```python
from build123d import *

# Parameters (mm, degrees)
BOSS_EXTRUDE1_DEPTH     = 6.35
CUT_EXTRUDE2_DEPTH      = 2.54
CUT_EXTRUDE2_DEPTH_BACK = 127
CUT_EXTRUDE4_DEPTH      = 127
CUT_EXTRUDE4_DEPTH_BACK = 127
CUT_EXTRUDE5_DEPTH      = 127
CUT_EXTRUDE5_DEPTH_BACK = 127


with BuildPart() as part:
    # Sketch1 → Boss-Extrude1 (new body)
    with BuildSketch(Plane.XY):
        Polygon((0, 0), (127, 0), (127, 101.6), (0, 101.6), (-70.692427737, 172.292427737), (-91.896861793, 151.087993682), (-91.896861793, 0), align=None)
    extrude(amount=BOSS_EXTRUDE1_DEPTH)

    # Sketch2 → Cut-Extrude2 (cut, two sides)
    with BuildSketch(Plane(origin=(0, 0, 0), x_dir=(-1, 0, 0), z_dir=(0, 0, -1))) as cut_extrude2_sk:
        Polygon((-61.321024484, 65.678975516), (-25.4, 101.6), (-31.75, 101.6), (-49.710512242, 83.639487758), (-67.671024484, 65.678975516), align=None)
    extrude(amount=CUT_EXTRUDE2_DEPTH, mode=Mode.SUBTRACT)
    extrude(cut_extrude2_sk.sketch, amount=-CUT_EXTRUDE2_DEPTH_BACK, mode=Mode.SUBTRACT)

    # Sketch3 → Cut-Extrude4 (cut, two sides)
    with BuildSketch(Plane(origin=(0, 0, 0), x_dir=(-1, 0, 0), z_dir=(0, 0, -1))) as cut_extrude4_sk:
        Polygon((-88.9, 101.6), (-101.6, 101.6), (-101.6, 98.425), (-96.5327, 98.425), (-96.5327, 85.725), (-93.9673, 85.725), (-93.9673, 98.425), (-88.9, 98.425), align=None)
        Polygon((-57.15, 101.6), (-69.85, 101.6), (-69.85, 98.425), (-64.77, 98.425), (-64.77, 85.725), (-62.23, 85.725), (-62.23, 98.425), (-57.15, 98.425), align=None)
        Polygon((-127, 82.55), (-127, 69.85), (-123.825, 69.85), (-123.825, 74.9173), (-111.125, 74.9173), (-111.125, 77.4827), (-123.825, 77.4827), (-123.825, 82.55), align=None)
        Polygon((-127, 57.15), (-127, 44.45), (-123.825, 44.45), (-123.825, 49.5173), (-111.125, 49.5173), (-111.125, 52.0827), (-123.825, 52.0827), (-123.825, 57.15), align=None)
        Polygon((-127, 31.75), (-127, 25.4), (-127, 19.05), (-123.825, 19.05), (-123.825, 24.1173), (-111.125, 24.1173), (-111.125, 26.6827), (-123.825, 26.6827), (-123.825, 31.75), align=None)
        Polygon((-101.6, 3.302), (-101.6, 0), (-88.9, 0), (-88.9, 3.302), (-93.9673, 3.302), (-93.9673, 16.002), (-96.5327, 16.002), (-96.5327, 3.302), align=None)
        Polygon((-25.4, 3.302), (-25.4, 0), (-12.7, 0), (-12.7, 3.302), (-17.7673, 3.302), (-17.7673, 16.002), (-20.3327, 16.002), (-20.3327, 3.302), align=None)
        Polygon((50.8, 3.302), (50.8, 0), (63.5, 0), (63.5, 3.302), (58.4327, 3.302), (58.4327, 16.002), (55.8673, 16.002), (55.8673, 3.302), align=None)
        Polygon((88.721861793, 31.42199842), (91.896861793, 31.42199842), (91.896861793, 44.12199842), (88.721861793, 44.12199842), (88.721861793, 39.05469842), (76.021861793, 39.05469842), (76.021861793, 36.48929842), (88.721861793, 36.48929842), align=None)
        Polygon((88.721861793, 69.193996841), (91.896861793, 69.193996841), (91.896861793, 81.893996841), (88.721861793, 81.893996841), (88.721861793, 76.826696841), (76.021861793, 76.826696841), (76.021861793, 74.261296841), (88.721861793, 74.261296841), align=None)
        Polygon((88.721861793, 106.965995261), (91.896861793, 106.965995261), (91.896861793, 119.665995261), (88.721861793, 119.665995261), (88.721861793, 114.598695261), (76.021861793, 114.598695261), (76.021861793, 112.033295261), (88.721861793, 112.033295261), align=None)
        Polygon((70.692427737, 158.822043556), (66.202299677, 154.331915495), (63.957235647, 156.576979525), (68.447363707, 161.067107586), align=None)
    extrude(amount=CUT_EXTRUDE4_DEPTH, mode=Mode.SUBTRACT)
    extrude(cut_extrude4_sk.sketch, amount=-CUT_EXTRUDE4_DEPTH_BACK, mode=Mode.SUBTRACT)

    # Sketch4 → Cut-Extrude5 (cut, two sides)
    with BuildSketch(Plane.XY) as cut_extrude5_sk:
        Polygon((-81.917747889, 147.596723404), (-79.672683858, 149.841787435), (-75.182555798, 145.351659374), (-77.427619828, 143.106595344), align=None)
    extrude(amount=CUT_EXTRUDE5_DEPTH, mode=Mode.SUBTRACT)
    extrude(cut_extrude5_sk.sketch, amount=-CUT_EXTRUDE5_DEPTH_BACK, mode=Mode.SUBTRACT)


solid = part.part
```
Model file for the job. Use its own axes, mm. A direction names the side the tool comes from. Coordinates: 2 decimals unless noted, no trailing zeros. Order: outer loops, then holes, each group sorted by start corner. A loop starts at its lowest first (then second) coordinate and runs counter-clockwise, first axis right, second up. Notation, with made-up numbers: (63.25, 46) -> (79.25, 46) arc R19 cw to (79.25, 62) -> close; hole circle Ø9 at (-15.5, -26.75). An arc over 180 degrees is marked (long way). Return JSON: item names as keys, results as strings.
Item 1: Slice it at B-B (x = 46.5). Write the cut outline in (y, z), then the cut area to 3 significant figures.
Model answer:
{"outline": "(0, 0) -> (80.5, 0) -> (80.5, 6.35) -> (0, 6.35) -> close; (86.85, 0) -> (101.6, 0) -> (101.6, 6.35) -> (86.85, 6.35) -> close", "area": "605 mm²"}
Item 2: Slice it at A-A (y = 95). Write the cut outline in (x, z), then the cut area to 3 significant figures.
Model answer:
{"outline": "(-91.9, 0) -> (32, 0) -> (32, 6.35) -> (-91.9, 6.35) -> close; (38.35, 0) -> (62.23, 0) -> (62.23, 6.35) -> (38.35, 6.35) -> close; (64.77, 0) -> (93.97, 0) -> (93.97, 6.35) -> (64.77, 6.35) -> close; (96.53, 0) -> (127, 0) -> (127, 6.35) -> (96.53, 6.35) -> close", "area": "1,320 mm²"}
Item 3: Slice it at D-D (x = -13). Write the cut outline in (y, z), then the cut area to 3 significant figures.
Model answer:
{"outline": "(0, 0) -> (114.6, 0) -> (114.6, 6.35) -> (0, 6.35) -> close", "area": "728 mm²"}
Item 4: Pin check, flat tips, straight feed: P1, Ø1.5, axis at x = 98.5, z = 3, coming from the -Y side; P2, Ø1.6, axis at x = -90, z = 4, coming from the +Y side; P3, Ø2.5, axis at x = -90, z = 4.5, coming from the +Y side; P4, Ø5, axis at x = -44, y = 19, coming from the -Z side. Stop position of each tip, or through.
Model answer:
{"P1": "stops at y = 3.3", "P2": "stops at y = 153.78", "P3": "stops at y = 154.23", "P4": "stops at z = 0"}
Item 5: Slice it at C-C (z = 2.25). Count the separate pieces of the cut face and the enclosed holes in it, then the cut area to 3 significant figures.
Model answer:
{"separate pieces": "1", "enclosed holes": "2", "area": "24,900 mm²"}
Item 6: 3-axis set-ups, long thin cutter, end or side, ignore diameter. For faces 1 (the face through (-82, 74.261, 3)), 2 (the face through (123.825, 29, 3)), 3 (the face through (91, 98.425, 3)): which of +Z, -Z, +X, -X, +Y, -Y reach the whole face in a straight line?
Model answer:
{"face 1": "+Z, -Z, -X", "face 2": "+Z, -Z, +X", "face 3": "+Z, -Z, +Y"}
Item 7: Wall check: line 1 along X through (y, z) = (13.5, 0.5); line 2 along Y through (x, z) = (115, 4.25); line 3 along X through (y, z) = (49, 5.5) (3 decimals). Give the ranges that are in metal, low to high. Write a range as from..to.
Model answer:
{"line 1": "x = -91.9..-58.43, -55.87..17.77, 20.33..93.97, 96.53..127", "line 2": "y = 0..24.12, 26.68..49.52, 52.08..74.92, 77.48..101.6", "line 3": "x = -91.897..123.825"}
